Here's how the part is built. I have some questions about the finished solid (model axes, mm). A direction names the side the tool comes from. Give positions to 0.01 mm unless a question says otherwise; leave off trailing zeros. Write each loop counter-clockwise with the first axis right and the second up, starting at its lowest first coordinate (ties: lowest second). Pieces come first, ordered by that corner, then holes. Notation, with made-up numbers: M 62,-2 L 116,-2 A27 ccw 116,23 Z; hole C 54.25,8 d11. An arc over 180 degrees is marked long. Answer as CSV lines item,"result". Start each with the question number.
Q1. Suppose I cut it at D-D (z = -12). Write out the boundary of the cut face in (x, y).
Q2. On a 3-axis mill with a long thin cutter (end or side, diameter ignored), from which of +Z, -Z, +X, -X, +Y, -Y can I reach the whole of each face in a straight line? I mean faces 1 (the flat face through (14, 2, -18.223)), 2 (the cylindrical face through (20, 2, -12)), 3 (the flat face through (14, 2.5, -14)), 4 (the flat face through (14, 2, -9.728)). Say none if no direction works.
Q3. Suppose I cut it at A-A (x = 24). Write out the boundary of the cut face in (y, z).
Q4. Suppose I cut it at B-B (z = -16.5). Write out the boundary of the cut face in (x, y).
Q5. If I drill on line 1 along Y through (x, z) = (23, -4.75); line 2 along Y through (x, z) = (16.5, -10.75); line 3 along X through (y, z) = (1.65, -10), over which ranges is the centre line in solid material (lowest first)?
Q6. Thinking about a two-plate mould opening in X: for faces 5 (the flat face through (18.262, 2, -14)), 6 (the flat face through (15, 1, -23)), 7 (the flat face through (0, 1, -11)), 8 (the flat face through (30, 1, -11)), which applies, +X half, -X half, draft (parallel to the pull), parting line (faces both ways), or undercut?
Q7. For pin 1 (1.1 mm diameter, centred on y = 2, z = -14.5, fed in from -X); pin 2 (6 mm diameter, centred on x = 9, z = -11, fed in from +Y); pin 3 (4 mm diameter, centred on x = 17, z = -4.5, fed in from +Y); pin 4 (2 mm diameter, centred on x = 23.5, y = 4, fed in from -Z), each with a flat end and sliding along its axis, tell me the tip position at first contact or that it passes through.
Q8. Suppose I cut it at C-C (y = 2.9). Write out the boundary of the cut face in (x, z), then the cut area to 3 significant figures.
```python
from build123d import *

# Parameters (mm, degrees)
ESBO_O1_W                = 30
ESBO_O1_H                = 23
RESSALTO_EXTRUS_O1_DEPTH = 1.5
ESBO_O2_W                = 8.558282237
ESBO_O2_H                = 8.494651886
RESSALTO_EXTRUS_O2_DEPTH = 1
ESBO_O3_R                = 4
RESSALTO_EXTRUS_O3_DEPTH = 3
FILETE1_R                = 1


with BuildPart() as part:
    # Esboço1 → Ressalto-extrusão1 (new body)
    with BuildSketch(Plane(origin=(0, 0, 0), x_dir=(1, 0, 0), z_dir=(0, 1, 0))):
        with Locations((15, 11.5)):
            Rectangle(ESBO_O1_W, ESBO_O1_H)
    extrude(amount=RESSALTO_EXTRUS_O1_DEPTH)

    # Esboço2 → Ressalto-extrusão2 (add)
    with BuildSketch(Plane(origin=(0, 1.5, 0), x_dir=(-1, 0, 0), z_dir=(0, 1, 0))):
        with Locations((-13.983300564, -13.975214048)):
            Rectangle(ESBO_O2_W, ESBO_O2_H)
    extrude(amount=RESSALTO_EXTRUS_O2_DEPTH)

    # Esboço3 → Ressalto-extrusão3 (add)
    with BuildSketch(Plane(origin=(0, 1.5, 0), x_dir=(1, 0, 0), z_dir=(0, 1, 0))):
        with Locations((24, 12)):
            Circle(ESBO_O3_R)
    extrude(amount=RESSALTO_EXTRUS_O3_DEPTH)

    # Filete1
    filete1_edges = [part.edges().sort_by_distance(p)[0] for p in [
        (20, 4.5, -12),
    ]]
    fillet(filete1_edges, radius=FILETE1_R)


solid = part.part
```
Resolved:
1,outline,"M 0,0 L 30,0 L 30,1.5 L 28,1.5 L 28,3.5 A1 ccw 27,4.5 L 21,4.5 A1 ccw 20,3.5 L 20,1.5 L 18.26,1.5 L 18.26,2.5 L 9.7,2.5 L 9.7,1.5 L 0,1.5 Z"
2,face 1,"-Z, +X, -X, +Y"
2,face 2,"+Y"
2,face 3,"+Z, -Z, -X, +Y"
2,face 4,"+Z, -X, +Y"
3,outline,"M 0,-23 L 1.5,-23 L 1.5,-16 L 3.5,-16 A1 ccw 4.5,-15 L 4.5,-9 A1 ccw 3.5,-8 L 1.5,-8 L 1.5,0 L 0,0 Z"
4,outline,"M 0,0 L 30,0 L 30,1.5 L 18.26,1.5 L 18.26,2.5 L 9.7,2.5 L 9.7,1.5 L 0,1.5 Z"
5,line 1,"0 to 1.5"
5,line 2,"0 to 2.5"
5,line 3,"9.7 to 18.26, 20.54 to 27.46"
6,face 5,"undercut"
6,face 6,"draft"
6,face 7,"-X half"
6,face 8,"+X half"
7,pin 1,"x = 0"
7,pin 2,"y = 2.5"
7,pin 3,"y = 1.5"
7,pin 4,"z = -16"
8,outline,"C 24,-12 d8"
8,area,"50.3 mm^2"
